For this review, take the finished solid that the model builds, in its own axes (mm). Face numbers are marked on the shaded views. A direction names the side the tool comes from. Round coordinates to 2 decimals unless told otherwise and drop trailing zeros. Loops run counter-clockwise (first coordinate to the right, second up) from the corner with the lowest first, then second, coordinate; pieces in that order, holes last.
1) Tool access review of the marked faces 4, 5 and 6: name each direction out of +Z, -Z, +X, -X, +Y, -Y from which nothing blocks a thin tool from reaching the whole face with its end or side.
2) Take a section at D-D (y = 49). State the section outline as (x, z) points.
3) Take a section at B-B (y = 28). State the section outline as (x, z) points.
4) Mouldability with a two-part tool opening along Y and no side actions: class the marked faces 1, 2 and 3 as pulls with the +Y half, pulls with the -Y half, needs draft (parallel to the pull), parting line crosses it, or undercut.
5) Wall thickness on L1, parallel to Y at x = -1.5, z = -2.5; L2, parallel to Y at x = 5.5, z = -7; L3, parallel to Y at x = 2.5, z = 15: over which ranges is each line inside the solid? List them lowest first.
6) Insertion check: pin 1 (12 mm diameter, centred on x = -2.5, y = 37.5, fed in from -Z) (3 decimals); pin 2 (3 mm diameter, centred on x = 0.5, z = 5, fed in from +Y); pin 3 (3 mm diameter, centred on x = -14, z = 3, fed in from +Y). Each pin has a flat end and moves straight along its axis. Give the tip position at first contact, or say it passes through.
7) Take a section at C-C (z = 15.5). State the section outline as (x, y) points.
8) Take a section at A-A (z = 0). State the section outline as (x, y) points (3 decimals), then the cut area to 3 significant figures.
```python
from build123d import *

# Parameters (mm, degrees)
SKETCH1_R           = 20.65
BOSS_EXTRUDE1_DEPTH = 5.98
SKETCH2_R           = 4
BOSS_EXTRUDE2_DEPTH = 23.4
BOSS_EXTRUDE3_DEPTH = 1.95
SKETCH4_R           = 4.375
BOSS_EXTRUDE4_DEPTH = 10.2
SKETCH5_R           = 3.165
BOSS_EXTRUDE5_DEPTH = 6.4
SKETCH6_R           = 2.1
BOSS_EXTRUDE6_DEPTH = 8


with BuildPart() as part:
    # Sketch1 → Boss-Extrude1 (new body)
    with BuildSketch(Plane(origin=(0, 0, 0), x_dir=(1, 0, 0), z_dir=(0, 1, 0))):
        Circle(SKETCH1_R)
    extrude(amount=BOSS_EXTRUDE1_DEPTH)

    # Sketch2 → Boss-Extrude2 (add)
    with BuildSketch(Plane(origin=(0, 5.98, 0), x_dir=(1, 0, 0), z_dir=(0, 1, 0))):
        with Locations((0, -16.65)):
            Circle(SKETCH2_R)
        with Locations((0, 16.65)):
            Circle(SKETCH2_R)
    extrude(amount=BOSS_EXTRUDE2_DEPTH)

    # Sketch3 → Boss-Extrude3 (add)
    with BuildSketch(Plane(origin=(0, 29.38, 0), x_dir=(1, 0, 0), z_dir=(0, 1, 0))):
        with BuildLine():
            Line((-4, -21.05), (4, -21.05))
            ThreePointArc((4, -21.05), (4.707106781, -20.757106781), (5, -20.05))
            Line((5, -20.05), (5, 20.05))
            ThreePointArc((5, 20.05), (4.707106781, 20.757106781), (4, 21.05))
            Line((4, 21.05), (-4, 21.05))
            ThreePointArc((-4, 21.05), (-4.707106781, 20.757106781), (-5, 20.05))
            Line((-5, 20.05), (-5, -20.05))
            ThreePointArc((-5, -20.05), (-4.707106781, -20.757106781), (-4, -21.05))
        make_face()
    extrude(amount=BOSS_EXTRUDE3_DEPTH)

    # Sketch4 → Boss-Extrude4 (add)
    with BuildSketch(Plane(origin=(0, 31.33, 0), x_dir=(1, 0, 0), z_dir=(0, 1, 0))):
        Circle(SKETCH4_R)
    extrude(amount=BOSS_EXTRUDE4_DEPTH)

    # Sketch5 → Boss-Extrude5 (add)
    with BuildSketch(Plane(origin=(0, 41.53, 0), x_dir=(1, 0, 0), z_dir=(0, 1, 0))):
        Circle(SKETCH5_R)
    extrude(amount=BOSS_EXTRUDE5_DEPTH)

    # Sketch6 → Boss-Extrude6 (add)
    with BuildSketch(Plane(origin=(0, 47.93, 0), x_dir=(1, 0, 0), z_dir=(0, 1, 0))):
        Circle(SKETCH6_R)
    extrude(amount=BOSS_EXTRUDE6_DEPTH)


solid = part.part
```
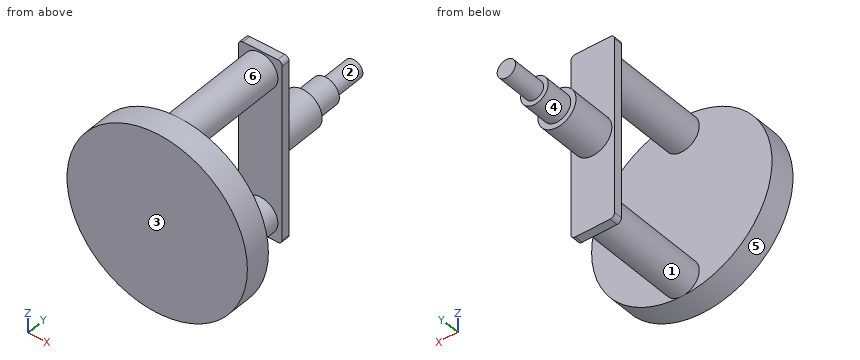
Response:
1. face 4: +Y
1. face 5: -Y
1. face 6: none
2. outline: circle Ø4.2 at (0, 0)
3. outline: circle Ø8 at (0, -16.65); circle Ø8 at (0, 16.65)
4. face 1: undercut
4. face 2: needs draft
4. face 3: pulls with the -Y half
5. L1: y = 0 to 5.98, 29.38 to 47.93
5. L2: y = 0 to 5.98
5. L3: y = 0 to 31.33
6. pin 1: stops at z = -4.375
6. pin 2: stops at y = 41.53
6. pin 3: stops at y = 5.98
7. outline: (-13.64, 0) - (13.64, 0) - (13.64, 5.98) - (3.83, 5.98) - (3.83, 29.38) - (5, 29.38) - (5, 31.33) - (-5, 31.33) - (-5, 29.38) - (-3.83, 29.38) - (-3.83, 5.98) - (-13.64, 5.98) - close
8. outline: (-20.65, 0) - (20.65, 0) - (20.65, 5.98) - (-20.65, 5.98) - close; (-5, 29.38) - (5, 29.38) - (5, 31.33) - (4.375, 31.33) - (4.375, 41.53) - (3.165, 41.53) - (3.165, 47.93) - (2.1, 47.93) - (2.1, 55.93) - (-2.1, 55.93) - (-2.1, 47.93) - (-3.165, 47.93) - (-3.165, 41.53) - (-4.375, 41.53) - (-4.375, 31.33) - (-5, 31.33) - close
8. area: 430 mm2
